```python
from build123d import *

# Parameters (mm, degrees)
F0_R     = 0.6
F1_DEPTH = 20
F2_W     = 18
F2_H     = 5
F2_W_2   = 2
F3_DEPTH = 4
F4_R     = 1
F5_DEPTH = 4


with BuildPart() as f1:
    # F0 (on Top) → F1 (new body)
    with BuildSketch(Plane.XY):
        with BuildLine():
            ThreePointArc((-2.085665, 0.7), (2.2, 0), (-2.085665, -0.7))
            Line((-2.085665, -0.7), (-3.7, -0.7))
            Line((-3.7, -0.7), (-3.7, -3.7))
            Line((-3.7, -3.7), (3.7, -3.7))
            Line((3.7, -3.7), (3.7, -1.4))
            Line((3.7, -1.4), (21.7, -1.4))
            ThreePointArc((21.7, -1.4), (23.114214, -0.814214), (23.7, 0.6))
            ThreePointArc((23.7, 0.6), (23.114214, 2.014214), (21.7, 2.6))
            Line((21.7, 2.6), (3.7, 2.6))
            Line((3.7, 2.6), (3.7, 3.7))
            Line((3.7, 3.7), (-3.7, 4.9))
            Line((-3.7, 4.9), (-3.7, 0.7))
            Line((-3.7, 0.7), (-2.085665, 0.7))
        make_face()
        with Locations((21.7, 0.6)):
            Circle(F0_R, mode=Mode.SUBTRACT)
    extrude(amount=F1_DEPTH)

    # F2 (on face) → F3 (cut)
    with BuildSketch(Plane.XZ.offset(1.4)):
        with Locations((12.7, 2.5)):
            Rectangle(F2_W, F2_H)
        with Locations((22.7, 2.5)):
            Rectangle(F2_W_2, F2_H)
        with Locations((22.7, 17.5)):
            Rectangle(F2_W_2, F2_H)
        with Locations((12.7, 17.5)):
            Rectangle(F2_W, F2_H)
    extrude(amount=-F3_DEPTH, mode=Mode.SUBTRACT)

    # F4 (on face) → F5 (cut)
    with BuildSketch(Plane(origin=(0, 2.6, 0), x_dir=(-1, 0, 0), z_dir=(0, 1, 0))):
        with Locations((-8.2, 10)):
            Circle(F4_R)
    extrude(amount=-F5_DEPTH, mode=Mode.SUBTRACT)


solid = f1.part
```
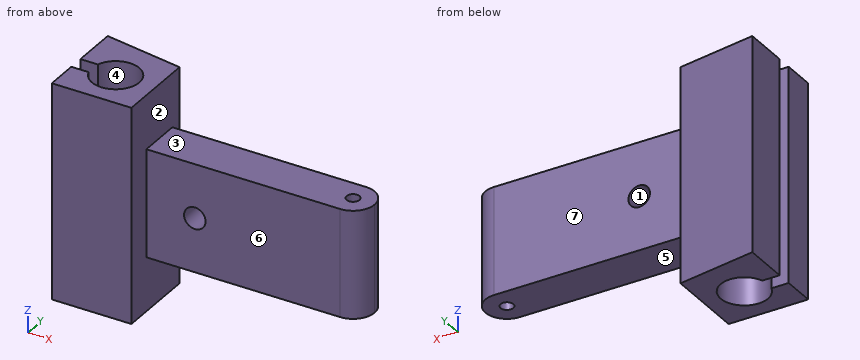
Read the model definition and answer for the solid it produces. Units are mm, in the model's axes. Face numbers are marked on the shaded views. A direction names the side the tool comes from. Coordinates: 2 decimals unless noted, no trailing zeros. Loops run counter-clockwise (first coordinate to the right, second up) from the corner with the lowest first, then second, coordinate; pieces in that order, holes last. Notation, with made-up numbers: (-20.75, -31.5) -> (23.25, -31.5) arc R9 ccw to (23.25, -16.5) -> close; hole circle Ø7 at (-7.75, -26). An arc over 180 degrees is marked (long way). Return JSON: item names as keys, results as strings.
Item 1: Find the intervals of material crossed by probe 1 along Y at (x, z) = (21.7, 11.75); probe 2 along Z at (x, y) = (8.25, 2.5); probe 3 along X at (y, z) = (-2.75, 6.75), in increasing order.
Answers:
{"probe 1": "y = -1.4 to 0, 1.2 to 2.6", "probe 2": "z = 5 to 9, 11 to 15", "probe 3": "x = -3.7 to 3.7"}
Item 2: Find section B-B (z = 10). Determine the outline of the cut face in (x, y), plus the area to 3 significant figures.
Answers:
{"outline": "(-3.7, -3.7) -> (3.7, -3.7) -> (3.7, -1.4) -> (7.2, -1.4) -> (7.2, 2.6) -> (3.7, 2.6) -> (3.7, 3.7) -> (-3.7, 4.9) -> (-3.7, 0.7) -> (-2.09, 0.7) arc R2.2 cw (long way) to (-2.09, -0.7) -> (-3.7, -0.7) -> close; (9.2, -1.4) -> (21.7, -1.4) arc R2 ccw to (23.7, 0.6) arc R2 ccw to (21.7, 2.6) -> (9.2, 2.6) -> close; hole circle Ø1.2 at (21.7, 0.6)", "area": "111 mm2"}
Item 3: Flat-ended cylindrical pins translate along their axes: P1, Ø1.6, axis at x = 21.7, y = 0.6, coming from the +Z side; P2, Ø8, axis at x = 11.5, z = 9.5, coming from the +Y side; P3, Ø1.2, axis at x = 8.2, z = 10, coming from the -Y side; P4, Ø3, axis at x = 13, y = 1, coming from the -Z side. Find the tip coordinate at first contact, or state that the pin passes through.
Answers:
{"P1": "stops at z = 15", "P2": "stops at y = 2.6", "P3": "passes through", "P4": "stops at z = 5"}
Item 4: For the marked faces 5, 6 and 7, determine the directions among +Z, -Z, +X, -X, +Y, -Y from which every point of the face is accessible in a straight line to the end or side of a thin tool.
Answers:
{"face 5": "-Z, +X, +Y, -Y", "face 6": "+Z, -Z, +X, -Y", "face 7": "+Z, -Z, +X, +Y"}
Item 5: For a pull along X with two mould halves and no side action, classify the marked faces 1, 2, 3 and 4 as +X half, -X half, draft (parallel to the pull), parting line (faces both ways), or undercut.
Answers:
{"face 1": "undercut", "face 2": "+X half", "face 3": "draft", "face 4": "undercut"}
Item 6: Find section C-C (z = 5.75). Determine the outline of the cut face in (x, y), plus the area to 3 significant figures.
Answers:
{"outline": "(-3.7, -3.7) -> (3.7, -3.7) -> (3.7, -1.4) -> (21.7, -1.4) arc R2 ccw to (23.7, 0.6) arc R2 ccw to (21.7, 2.6) -> (3.7, 2.6) -> (3.7, 3.7) -> (-3.7, 4.9) -> (-3.7, 0.7) -> (-2.09, 0.7) arc R2.2 cw (long way) to (-2.09, -0.7) -> (-3.7, -0.7) -> close; hole circle Ø1.2 at (21.7, 0.6)", "area": "119 mm2"}
Item 7: Find section D-D (y = -1). Determine the outline of the cut face in (x, z).
Answers:
{"outline": "(-3.7, 0) -> (-1.96, 0) -> (-1.96, 20) -> (-3.7, 20) -> close; (1.96, 0) -> (3.7, 0) -> (3.7, 5) -> (22.9, 5) -> (22.9, 15) -> (3.7, 15) -> (3.7, 20) -> (1.96, 20) -> close; hole circle Ø2 at (8.2, 10)"}
Item 8: Find section A-A (x = 8.2). Determine the outline of the cut face in (y, z).
Answers:
{"outline": "(-1.4, 5) -> (2.6, 5) -> (2.6, 9) -> (-1.4, 9) -> close; (-1.4, 11) -> (2.6, 11) -> (2.6, 15) -> (-1.4, 15) -> close"}
